Part model, mm, in its own coordinate system. A direction names the side the tool comes from. Coordinates: 2 decimals unless noted, no trailing zeros. Loops run counter-clockwise (first coordinate to the right, second up) from the corner with the lowest first, then second, coordinate; pieces in that order, holes last. Notation, with made-up numbers: (10, 71.5) - (38, 71.5) arc R31 ccw to (38, 96.5) - close; hole circle Ø11 at (67, 67). An arc over 180 degrees is marked (long way). Answer as CSV lines item,"result".
from build123d import *

# Parameters (mm, degrees)
SKETCH1_W            = 180
SKETCH1_H            = 79
BOSS_EXTRUDE1_DEPTH  = 5
FILLET1_R            = 5
SKETCH2_W            = 3
SKETCH2_H            = 8
BOSS_EXTRUDE2_DEPTH  = 4.5
FILLET2_R            = 2
SKETCH3_R            = 1.25
BOSS_EXTRUDE3_DEPTH  = 8
LPATTERN1_COUNT      = 2
LPATTERN1_PITCH      = 50
LPATTERN1_COUNT_DIR2 = 2
LPATTERN1_PITCH_DIR2 = 174.9
SKETCH4_W            = 83
SKETCH4_H            = 22
CUT_EXTRUDE1_DEPTH   = 2
SKETCH5_W            = 77
SKETCH5_H            = 16
CUT_EXTRUDE2_DEPTH   = 3


with BuildPart() as part:
    # Sketch1 → Boss-Extrude1 (new body)
    with BuildSketch(Plane.XY):
        Rectangle(SKETCH1_W, SKETCH1_H)
    extrude(amount=BOSS_EXTRUDE1_DEPTH)

    # Fillet1
    fillet1_edges = [part.edges().sort_by_distance(p)[0] for p in [
        (90, 0, 0),
    ]]
    fillet(fillet1_edges, radius=FILLET1_R - 0.0001)  # a hair under: the kernel refuses the full size

    # Sketch2 → Boss-Extrude2 (add)
    with BuildSketch(Plane.XY.offset(5)):
        with Locations((-88.5, -24.5)):
            Rectangle(SKETCH2_W, SKETCH2_H)
        with Locations((-88.5, 25.5)):
            Rectangle(SKETCH2_W, SKETCH2_H)
        with Locations((83.4, 25.5)):
            Rectangle(SKETCH2_W, SKETCH2_H)
        with Locations((83.4, -24.5)):
            Rectangle(SKETCH2_W, SKETCH2_H)
    extrude(amount=BOSS_EXTRUDE2_DEPTH)

    # Fillet2
    fillet2_edges = [part.edges().sort_by_distance(p)[0] for p in [
        (-87, -24.5, 9.5),
        (-87, 25.5, 9.5),
        (81.9, 25.5, 9.5),
        (81.9, -24.5, 9.5),
    ]]
    fillet(fillet2_edges, radius=FILLET2_R)

    # Sketch3 → Boss-Extrude3 (add)
    with BuildSketch(Plane(origin=(0, 29.5, 0), x_dir=(1, 0, 0), z_dir=(0, 1, 0))):
        with Locations((84.9, -8.25)):
            Circle(SKETCH3_R)
    boss_extrude3 = extrude(amount=-BOSS_EXTRUDE3_DEPTH)

    # LPattern1: Boss-Extrude3 2 × 2
    with Locations(*[(-j * LPATTERN1_PITCH_DIR2, -i * LPATTERN1_PITCH, 0) for i in range(LPATTERN1_COUNT) for j in range(LPATTERN1_COUNT_DIR2) if (i, j) != (0, 0)]):
        add(boss_extrude3)

    # Sketch4 → Cut-Extrude1 (cut)
    with BuildSketch(Plane.XY.offset(5)):
        Rectangle(SKETCH4_W, SKETCH4_H)
    extrude(amount=-CUT_EXTRUDE1_DEPTH, mode=Mode.SUBTRACT)

    # Sketch5 → Cut-Extrude2 (cut)
    with BuildSketch(Plane.XY.offset(3)):
        Rectangle(SKETCH5_W, SKETCH5_H)
    extrude(amount=-CUT_EXTRUDE2_DEPTH, mode=Mode.SUBTRACT)


solid = part.part
Q1. Wall check: L1, parallel to Y at x = -2.5, z = 3.25; L2, parallel to Y at x = 23.5, z = 1; L3, parallel to Z at x = -8, y = 15. Give the ranges that are in metal, low to high.
Results:
L1,"y = -39.5 to -11, 11 to 39.5"
L2,"y = -39.5 to -8, 8 to 39.5"
L3,"z = 0 to 5"
Q2. Which spindle directions (+Z, -Z, +X, -X, +Y, -Y) get a long thin tool onto all of the face, cutting with end or side? Do faces 4 (the face through (84, -28.5, 7)), 5 (the face through (-1, 8, 2)), 6 (the face through (-90, -1, 3)). Say none if no direction does.
Results:
face 4,"+Z, +X, -X, -Y"
face 5,"+Z, -Z"
face 6,"-Z, -X, +Y, -Y"
Q3. Saw through at C-C (x = 56). Give the cut face in (y, z).
Results:
outline,"(-39.5, 0) - (39.5, 0) - (39.5, 5) - (-39.5, 5) - close"
Q4. Saw through at B-B (x = -20). Give the cut face in (y, z), then the cut area to 3 significant figures.
Results:
outline,"(-39.5, 0) - (-8, 0) - (-8, 3) - (-11, 3) - (-11, 5) - (-39.5, 5) - close; (8, 0) - (39.5, 0) - (39.5, 5) - (11, 5) - (11, 3) - (8, 3) - close"
area,"303 mm^2"
Q5. Two-plate mould, pull along X, no slides. Class faces 1 (the face through (-89, 29.5, 7)), 2 (the face through (89, 1, 2)), 3 (the face through (38.5, 0, 2)): released by +X, released by -X, zero draft, split by the parting line, or undercut.
Results:
face 1,"zero draft"
face 2,"released by +X"
face 3,"undercut"
Q6. Flat gauge pins, fed straight in: pin 1 (3.5 mm diameter, centred on x = -88.5, z = 7, fed in from -Y); pin 2 (1.2 mm diameter, centred on y = 27, z = 6, fed in from +X); pin 3 (3.5 mm diameter, centred on x = -89.5, z = 7.5, fed in from +Y); pin 4 (1.5 mm diameter, centred on x = 18.5, y = -5.5, fed in from -Z). Where does each tip first touch, or does it go through?
Results:
pin 1,"stops at y = -28.5"
pin 2,"stops at x = 84.9"
pin 3,"stops at y = 29.5"
pin 4,"passes through"
